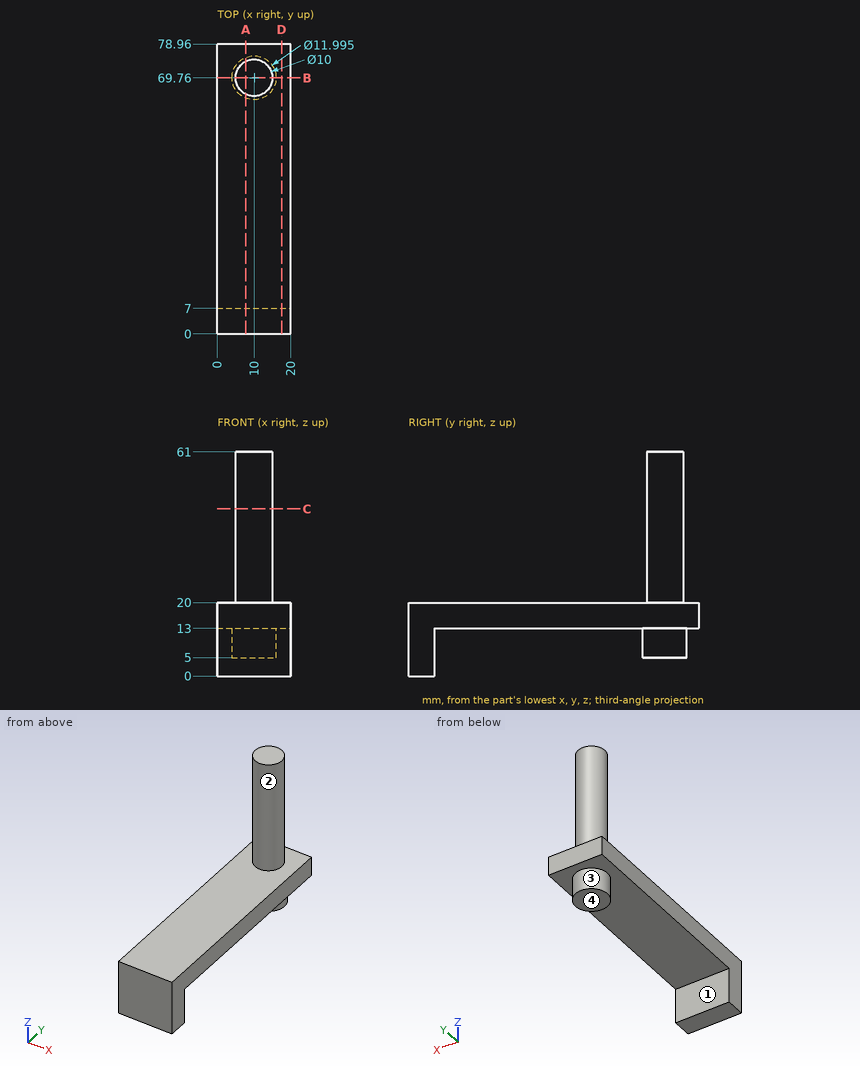
Can you work these out from the drawing? Everything is in mm from the part's minimum corner. A direction names the side the tool comes from. Give positions to 0.01 mm unless a question says otherwise; leave off trailing zeros. Loops run counter-clockwise (first coordinate to the right, second up) from the corner with the lowest first, then second, coordinate; pieces in that order, holes last. Notation, with made-up numbers: M 83.25,68.25 L 114.25,68.25 A14 cw 114.25,85.25 Z; hole C 34.5,89 d4. An arc over 180 degrees is marked long. Use CSV: the item, a comma, the result in double quotes. Start each with the question number.
1. Imagine slicing it at D-D, the plane x = 17.5. Write out the boundary of the cut face in (y, z).
2. Imagine slicing it at B-B, the plane y = 69.76. Write out the boundary of the cut face in (x, z).
3. If I drill on L1, parallel to Z at x = 14.75, y = 52; L2, parallel to Y at x = 10, z = 29; L3, parallel to Z at x = 10, y = 73.5, over which ranges is the centre line in solid material (lowest first)?
4. For P1, Ø1.5, axis at x = 11.5, y = 18.5, coming from the -Z side; P2, Ø6, axis at x = 7.5, y = 25, coming from the +Z side; P3, Ø1.5, axis at x = 16.5, z = 50, coming from the -Y side; P4, Ø9.5, axis at x = 9.5, y = 69.5, coming from the -Z side, each with a flat end and sliding along its axis, tell me the tip position at first contact or that it passes through.
5. Imagine slicing it at A-A, the plane x = 7.75. Write out the boundary of the cut face in (y, z) (1 decimal).
6. Imagine slicing it at C-C, the plane z = 45.5. Write out the boundary of the cut face in (x, y).
7. On a 3-axis mill with a long thin cutter (end or side, diameter ignored), from which of +Z, -Z, +X, -X, +Y, -Y can I reach the whole of each face in a straight line? I mean the marked faces 1, 2, 3 and 4. Say none if no direction works.
Response values:
1,outline,"M 0,0 L 7,0 L 7,13 L 78.96,13 L 78.96,20 L 0,20 Z"
2,outline,"M 0,13 L 4,13 L 4,5 L 16,5 L 16,13 L 20,13 L 20,20 L 15,20 L 15,61 L 5,61 L 5,20 L 0,20 Z"
3,L1,"13 to 20"
3,L2,"64.76 to 74.76"
3,L3,"5 to 61"
4,P1,"z = 13"
4,P2,"z = 20"
4,P3,"through"
4,P4,"z = 5"
5,outline,"M 0,0 L 7,0 L 7,13 L 64.2,13 L 64.2,5 L 75.3,5 L 75.3,13 L 79,13 L 79,20 L 74.2,20 L 74.2,61 L 65.3,61 L 65.3,20 L 0,20 Z"
6,outline,"C 10,69.76 d10"
7,face 1,"-Z, +X, -X"
7,face 2,"+Z"
7,face 3,"-Z"
7,face 4,"-Z, +X, -X, +Y"
